Source: CAD feature listing. Evaluate the final solid. Frame: model axes, mm. A direction names the side the tool comes from. Round coordinates to 2 decimals unless told otherwise and drop trailing zeros. Loops run counter-clockwise (first coordinate to the right, second up) from the corner with the lowest first, then second, coordinate; pieces in that order, holes last. Notation, with made-up numbers: (83, 34) - (96, 34) arc R18 cw to (96, 47) - close; hole circle Ø4 at (-36, -8.75). An arc over 180 degrees is marked (long way). Use CSV: the item, a comma, the result in double quotes. Start each with the question number.
from build123d import *

# Parameters (mm, degrees)
SKETCH1_W           = 200
SKETCH1_H           = 300
SKETCH1_W_2         = 135
SKETCH1_H_2         = 235
BOSS_EXTRUDE1_DEPTH = 5
SKETCH3_R           = 5
BOSS_EXTRUDE2_DEPTH = 10
SKETCH4_R           = 9
SKETCH4_R_2         = 8
CUT_EXTRUDE1_DEPTH  = 2
SKETCH5_R           = 0.5
CUT_EXTRUDE2_DEPTH  = 5
SKETCH6_R           = 1.5
CUT_EXTRUDE3_DEPTH  = 5


with BuildPart() as part:
    # Sketch1 → Boss-Extrude1 (new body)
    with BuildSketch(Plane(origin=(0, 0, 0), x_dir=(1, 0, 0), z_dir=(0, 1, 0))):
        Rectangle(SKETCH1_W, SKETCH1_H)
        Rectangle(SKETCH1_W_2, SKETCH1_H_2, mode=Mode.SUBTRACT)
    extrude(amount=BOSS_EXTRUDE1_DEPTH)

    # Sketch3 → Boss-Extrude2 (add)
    with BuildSketch(Plane(origin=(100, 0, 0), x_dir=(0, 0, -1), z_dir=(1, 0, 0))):
        with BuildLine():
            Line((-14, 5), (14, 5))
            Line((14, 5), (14, -7))
            ThreePointArc((14, -7), (0, -21.000001209), (-14, -7))
            Line((-14, -7), (-14, 5))
        make_face()
        with Locations((0, -9.127388195)):
            Circle(SKETCH3_R, mode=Mode.SUBTRACT)
    boss_extrude2 = extrude(amount=BOSS_EXTRUDE2_DEPTH)

    # Mirror1: Boss-Extrude2 across plane
    add(boss_extrude2.mirror(Plane(origin=(0, 0, 0), x_dir=(0, 0, 1), z_dir=(1, 0, 0))))

    # Sketch4 → Cut-Extrude1 (cut)
    with BuildSketch(Plane(origin=(0, 5, 0), x_dir=(1, 0, 0), z_dir=(0, 1, 0))):
        with Locations(Location((0, -139, 0), (0, 0, 270))):
            Circle(SKETCH4_R)
        with Locations(Location((0, -139, 0), (0, 0, 270))):
            Circle(SKETCH4_R_2, mode=Mode.SUBTRACT)
    cut_extrude1 = extrude(amount=-CUT_EXTRUDE1_DEPTH, mode=Mode.SUBTRACT)

    # Mirror2: Cut-Extrude1 across plane
    add(cut_extrude1.mirror(Plane.XY), mode=Mode.SUBTRACT)

    # Sketch5 → Cut-Extrude2 (cut)
    with BuildSketch(Plane(origin=(0, 5, 0), x_dir=(1, 0, 0), z_dir=(0, 1, 0))):
        with Locations(Location((0, -134, 0), (0, 0, 270))):
            Circle(SKETCH5_R)
        with Locations(Location((0, -144, 0), (0, 0, 270))):
            Circle(SKETCH5_R)
    cut_extrude2 = extrude(amount=-CUT_EXTRUDE2_DEPTH, mode=Mode.SUBTRACT)

    # Mirror3: Cut-Extrude2 across plane
    add(cut_extrude2.mirror(Plane.XY), mode=Mode.SUBTRACT)

    # Sketch6 → Cut-Extrude3 (cut)
    with BuildSketch(Plane(origin=(0, 5, 0), x_dir=(1, 0, 0), z_dir=(0, 1, 0))):
        with Locations(Location((-82.5, 6, 0), (0, 0, 270))):
            Circle(SKETCH6_R)
        with Locations(Location((-82.5, -6, 0), (0, 0, 270))):
            Circle(SKETCH6_R)
    cut_extrude3 = extrude(amount=-CUT_EXTRUDE3_DEPTH, mode=Mode.SUBTRACT)

    # Mirror4: Cut-Extrude3 across plane
    add(cut_extrude3.mirror(Plane(origin=(0, 0, 0), x_dir=(0, 0, 1), z_dir=(1, 0, 0))), mode=Mode.SUBTRACT)


solid = part.part
1. Line query: line 1 along Z through (x, y) = (82.5, 3.6); line 2 along Y through (x, z) = (104.25, 0); line 3 along X through (y, z) = (2.45, 6). Output: solid intervals per line, ascending.
2. Section query B-B on z = -60.5. Return the cut outline in (x, y), and give its area (3 significant figures).
3. Section query C-C on z = 139. Return the cut outline in (x, y).
4. Mould query, pull axis Z, two halves, no side actions, for faces 1 (the cylindrical face through (-104.93, -14.01, 1.08)), 2 (the flat face through (-100, -3, 0)), 3 (the cylindrical face through (105, -21, 0)). Classes: +Z half, -Z half, draft (parallel to the pull), parting line (faces both ways), or undercut.
5. Section query D-D on z = 0. Return the cut outline in (x, y).
6. Section query A-A on x = -61.5. Return the cut outline in (y, z), and give its area (3 significant figures).
7. Reachability of faces 4 (the flat face through (105, -1, -14)), 5 (the cylindrical face through (-3.06, 4.01, 146.39)), 6 (the flat face through (105, -1, 14)), 7 (the flat face through (-105, -1, -14)), 8 (the flat face through (-105, -1, 14)) from +Z, -Z, +X, -X, +Y, -Y: full face, straight path, thin tool, end or side. Return the list, or none.
8. Contact query for flat-ended pins moving along their axis: P1, Ø1.5, axis at y = 2, z = -16.5, coming from the +X side; P2, Ø6, axis at y = -9.13, z = 0, coming from the -X side; P3, Ø3.5, axis at x = 82.5, z = -6, coming from the -Y side; P4, Ø1.5, axis at y = 1.5, z = 107.5, coming from the -X side. Output: stop coordinate, or through.
Values:
1,line 1,"z = -150 to -7.5, -4.5 to 4.5, 7.5 to 150"
1,line 2,"y = -21 to -14.13, -4.13 to 5"
1,line 3,"x = -110 to -84, -81 to -67.5, 67.5 to 81, 84 to 110"
2,outline,"(-100, 0) - (-67.5, 0) - (-67.5, 5) - (-100, 5) - close; (67.5, 0) - (100, 0) - (100, 5) - (67.5, 5) - close"
2,area,"325 mm^2"
3,outline,"(-100, 0) - (100, 0) - (100, 5) - (9, 5) - (9, 3) - (8, 3) - (8, 5) - (-8, 5) - (-8, 3) - (-9, 3) - (-9, 5) - (-100, 5) - close"
4,face 1,"undercut"
4,face 2,"draft"
4,face 3,"parting line"
5,outline,"(-110, -21) - (-100, -21) - (-100, -14.13) - (-110, -14.13) - close; (-110, -4.13) - (-100, -4.13) - (-100, 0) - (-67.5, 0) - (-67.5, 5) - (-110, 5) - close; (67.5, 0) - (100, 0) - (100, -4.13) - (110, -4.13) - (110, 5) - (67.5, 5) - close; (100, -21) - (110, -21) - (110, -14.13) - (100, -14.13) - close"
6,outline,"(0, -150) - (5, -150) - (5, -117.5) - (0, -117.5) - close; (0, 117.5) - (5, 117.5) - (5, 150) - (0, 150) - close"
6,area,"325 mm^2"
7,face 4,"-Z, +X, +Y, -Y"
7,face 5,"+Y"
7,face 6,"+Z, +X, +Y, -Y"
7,face 7,"-Z, -X, +Y, -Y"
7,face 8,"+Z, -X, +Y, -Y"
8,P1,"stops at x = 100"
8,P2,"passes through"
8,P3,"stops at y = 0"
8,P4,"stops at x = -100"
